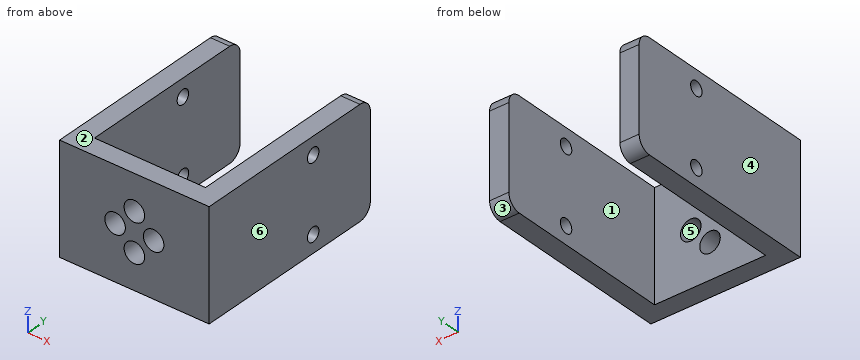
from build123d import *

# Parameters (mm, degrees)
SKETCH_1_W          = 17.3
SKETCH_1_H          = 17
SKETCH_1_R          = 1.6
EXTRUDE_1_DEPTH     = 3
SKETCH_2_W          = 3
SKETCH_2_H          = 17
EXTRUDE_2_DEPTH     = 31
FILLET_1_R          = 2
SKETCH_3_R          = 1.1
CUT_EXTRUDE_1_DEPTH = 28


with BuildPart() as part:
    # 草图1 → 凸台-拉伸1 (new body)
    with BuildSketch(Plane(origin=(0, 0, 0), x_dir=(1, 0, 0), z_dir=(0, 1, 0))):
        Rectangle(SKETCH_1_W, SKETCH_1_H)
        with Locations(Location((0, 3, 0), (0, 0, 270))):
            Circle(SKETCH_1_R, mode=Mode.SUBTRACT)
        with Locations(Location((3, 0, 0), (0, 0, 270))):
            Circle(SKETCH_1_R, mode=Mode.SUBTRACT)
        with Locations(Location((0, -3, 0), (0, 0, 90))):
            Circle(SKETCH_1_R, mode=Mode.SUBTRACT)
        with Locations(Location((-3, 0, 0), (0, 0, 90))):
            Circle(SKETCH_1_R, mode=Mode.SUBTRACT)
    extrude(amount=EXTRUDE_1_DEPTH)

    # 草图2 → 凸台-拉伸2 (add)
    with BuildSketch(Plane(origin=(0, 0, 0), x_dir=(1, 0, 0), z_dir=(0, 1, 0))):
        with Locations((10.15, 0)):
            Rectangle(SKETCH_2_W, SKETCH_2_H)
        with Locations((-10.15, 0)):
            Rectangle(SKETCH_2_W, SKETCH_2_H)
    extrude(amount=EXTRUDE_2_DEPTH)

    # 圆角1
    fillet_1_edges = [part.edges().sort_by_distance(p)[0] for p in [
        (-10.15, 31, -8.5),
        (-10.15, 31, 8.5),
        (10.15, 31, 8.5),
        (10.15, 31, -8.5),
    ]]
    fillet(fillet_1_edges, radius=FILLET_1_R)

    # 草图3 → 切除-拉伸1 (cut)
    with BuildSketch(Plane.ZY.offset(11.65)):
        with Locations((5.75, 20)):
            Circle(SKETCH_3_R)
        with Locations((-5.75, 20)):
            Circle(SKETCH_3_R)
    extrude(amount=-CUT_EXTRUDE_1_DEPTH, mode=Mode.SUBTRACT)


solid = part.part
Work out the finished part from the listing and answer in its coordinate system (mm). Face numbers are marked on the shaded views. A direction names the side the tool comes from. Give positions to 0.01 mm unless a question says otherwise; leave off trailing zeros. Order: outer loops, then holes, each group sorted by start corner. A loop starts at its lowest first (then second) coordinate and runs counter-clockwise, first axis right, second up. Notation, with made-up numbers: (-32, 33) -> (11, 33) arc R10 ccw to (11, 37) -> close; hole circle Ø3 at (84, 72.25). An arc over 180 degrees is marked (long way). Answer as a JSON object with one key per item and string values. Group by question number.
1. Consider line 1 along X through (y, z) = (0.85, 3); line 2 along Y through (x, z) = (10.25, -5.75); line 3 along X through (y, z) = (6, 6.75). Determine where each line is inside the solid, lowest interval first. Write a range as [from, to].
2. Section C-C on y = 7 is taken. Determine the outline of the cut face in (x, z), plus the area to 3 significant figures.
3. Section A-A on y = 20 is taken. Determine the outline of the cut face in (x, z).
4. The mould has two halves that part along X. Classify the marked faces 3, 4, 5 and 6: released by +X, released by -X, zero draft, split by the parting line, or undercut.
5. A tool of negligible diameter and unlimited length cuts with its end or side. For the marked faces 1 and 2, from which of +Z, -Z, +X, -X, +Y, -Y can it reach the whole face along a straight path? Write none if from no direction.
6. Flat-ended cylindrical pins translate along their axes: pin 1 Ø2 at (y, z) = (20, 5.75) entering from +X; pin 2 Ø4 at (x, z) = (0, 3) entering from +Y. Find the tip coordinate at first contact, or state that the pin passes through.
7. Section D-D on x = 0 is taken. Determine the outline of the cut face in (y, z).
8. Section B-B on x = -3 is taken. Determine the outline of the cut face in (y, z), plus the area to 3 significant figures.
Result sheet:
{
 "1": {"line 1": "x = [-11.65, -1.6], [1.6, 11.65]", "line 2": "y = [0, 18.9], [21.1, 31]", "line 3": "x = [-11.65, -8.65], [8.65, 11.65]"},
 "2": {"outline": "(-11.65, -8.5) -> (-8.65, -8.5) -> (-8.65, 8.5) -> (-11.65, 8.5) -> close; (8.65, -8.5) -> (11.65, -8.5) -> (11.65, 8.5) -> (8.65, 8.5) -> close", "area": "102 mm^2"},
 "3": {"outline": "(-11.65, -8.5) -> (-8.65, -8.5) -> (-8.65, -6.85) -> (-11.65, -6.85) -> close; (-11.65, -4.65) -> (-8.65, -4.65) -> (-8.65, 4.65) -> (-11.65, 4.65) -> close; (-11.65, 6.85) -> (-8.65, 6.85) -> (-8.65, 8.5) -> (-11.65, 8.5) -> close; (8.65, -8.5) -> (11.65, -8.5) -> (11.65, -6.85) -> (8.65, -6.85) -> close; (8.65, -4.65) -> (11.65, -4.65) -> (11.65, 4.65) -> (8.65, 4.65) -> close; (8.65, 6.85) -> (11.65, 6.85) -> (11.65, 8.5) -> (8.65, 8.5) -> close"},
 "4": {"face 3": "zero draft", "face 4": "released by -X", "face 5": "undercut", "face 6": "released by +X"},
 "5": {"face 1": "+Z, -Z, +Y", "face 2": "+Z, +X, -X, +Y, -Y"},
 "6": {"pin 1": "passes through", "pin 2": "stops at y = 3"},
 "7": {"outline": "(0, -8.5) -> (3, -8.5) -> (3, -4.6) -> (0, -4.6) -> close; (0, -1.4) -> (3, -1.4) -> (3, 1.4) -> (0, 1.4) -> close; (0, 4.6) -> (3, 4.6) -> (3, 8.5) -> (0, 8.5) -> close"},
 "8": {"outline": "(0, -8.5) -> (3, -8.5) -> (3, -1.6) -> (0, -1.6) -> close; (0, 1.6) -> (3, 1.6) -> (3, 8.5) -> (0, 8.5) -> close", "area": "41.4 mm^2"}
}
